The listing builds one solid part. Answer for the finished solid, in the listing's coordinates (mm). Face numbers are marked on the shaded views. A direction names the side the tool comes from. Coordinates: 2 decimals unless noted, no trailing zeros. Loops run counter-clockwise (first coordinate to the right, second up) from the corner with the lowest first, then second, coordinate; pieces in that order, holes last. Notation, with made-up numbers: M 55,-18.5 L 73,-18.5 A16 ccw 73,-0.5 Z; hole C 70,1.5 d4. An arc over 180 degrees is marked long. Answer as a JSON object with one key per item and string values. Group by question number.
1. A cutting plane is placed at C-C on z = 16. State how many separate pieces and enclosed holes the cut face has, and give its area (3 significant figures).
2. Straight lines are drawn through the part: L1, parallel to X at y = -4.5, z = 17; L2, parallel to X at y = -2.3, z = 17; L3, parallel to Z at x = 8, y = -1.95. For each, find the intervals that lie inside material, in ascending order.
3. A cutting plane is placed at A-A on z = 2.25. Give the vertices of the cut face in (x, y).
4. A cutting plane is placed at D-D on y = 7. Give the vertices of the cut face in (x, z).
5. A cutting plane is placed at B-B on x = 31. Give the vertices of the cut face in (y, z), and give its area (3 significant figures).
6. For the marked faces 1 and 2, determine the directions among +Z, -Z, +X, -X, +Y, -Y from which every point of the face is accessible in a straight line to the end or side of a thin tool.
7. Determine the mould class of the marked faces 3, 4, 5 and 6 for opening direction Y: released by +Y, released by -Y, zero draft, split by the parting line, or undercut.
8. Given pin 1 (3.5 mm diameter, centred on x = 46.52, z = 17, fed in from +Y); pin 2 (5 mm diameter, centred on x = 8, z = 17, fed in from +Y); pin 3 (1 mm diameter, centred on y = 9.5, z = 5, fed in from -X); pin 4 (7 mm diameter, centred on x = 46.52, z = 17, fed in from +Y), each flat-ended and moving along its own axis, determine where each tip first touches the part or whether it passes through.
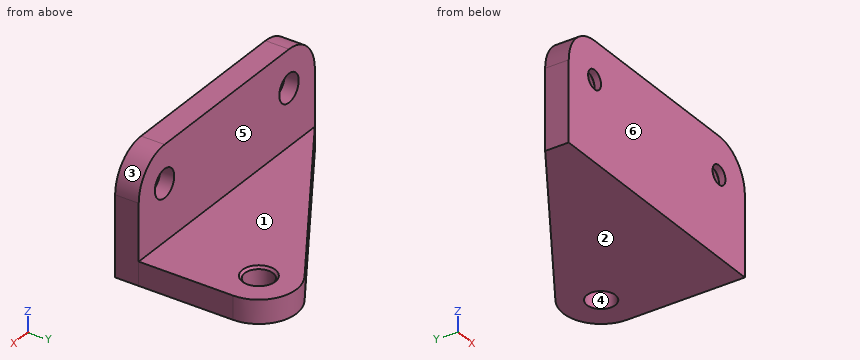
Autodesk Inventor part; units mm, degrees
ref_plane "YZ Plane" through (0, 0, 0) normal (1, 0, 0) x (0, 1, 0)
ref_plane "XZ Plane" through (0, 0, 0) normal (0, 1, 0) x (-1, 0, 0)
ref_plane "XY Plane" through (0, 0, 0) normal (0, 0, 1) x (1, 0, 0)
sketch "Boceto1" plane through (0, 0, 0) normal (0, 0, 1) x (1, 0, 0)
  circle A0 centre (46.519, 19.9996) radius 3
  arc A1 (54.519, 20) -> (42.2378, 26.7576) centre (46.519, 19.9996) ccw
  line L0 (54.52, 0) -> (54.519, 20)
  line L1 (0, 0) -> (42.2378, 26.7576)
  line L2 (0, 0) -> (0, -5)
  line L3 (0, -5) -> (54.52, -5)
  line L4 (54.52, -5) -> (54.52, 0)
  dimension "d5" = 50
  dimension "d6" = 20
  dimension "d8" = 5
  dimension "d9" = 54.52
extrude "Extrusión1" add sketch "Boceto1" along normal blind 5
sketch "Boceto2" plane through (0, 0, 5) normal (0, 0, 1) x (1, 0, 0)
  line L0 (0, 0) -> (0, -5)
  line L1 (0, 0) -> (0, -5)
  line L2 (0, -5) -> (54.52, -5)
  line L3 (0, -5) -> (54.52, -5)
  line L4 (54.52, -5) -> (54.52, 0)
  line L5 (54.52, -5) -> (54.52, 0)
  line L6 (54.52, 0) -> (0, 0)
extrude "Extrusión2" add sketch "Boceto2" along normal blind 20
fillet "Empalme1" radius 8 2 edges at (54.52, -2.5, 25) (0, -2.5, 25)
sketch "Boceto3" plane through (0, 0, 5) normal (0, 1, 0) x (1, 0, 0)
  circle A0 centre (8, -12) radius 3
  circle A1 centre (46.52, -12) radius 3
  point P0 (0, 5)
  dimension "d15" = 6
  dimension "d16" = 6
hole "Agujero1" at (8, 0, 17) at (46.52, 0, 17) direction (0, -1, 0) diameter 6 depth 3 tip angle 118
sketch "Boceto4" plane through (0, 0, 5) normal (0, 1, 0) x (1, 0, 0)
  circle A0 centre (8, -12) radius 3
  circle A1 centre (46.52, -12) radius 3
  point P0 (0, 5)
hole "Agujero2" at (46.52, 0, 17) at (8, 0, 17) direction (0, -1, 0) diameter 4 depth 5 tip angle 118
chamfer "Chaflán1" distance 0.5 angle 45 1 edges at (43.519, 19.9996, 5) measured on face at (33.1116, 5.8435, 5)
properties material "Cobre"
From the geometry:
{
 "1": {"separate pieces": "3", "enclosed holes": "0", "area": "223 mm²"},
 "2": {"L1": "x = 0 to 6, 10 to 44.52, 48.52 to 54.52", "L2": "x = 0 to 5, 11 to 43.52, 49.52 to 54.52", "L3": "z = 0 to 14, 20 to 25"},
 "3": {"outline": "M 0,-5 L 54.52,-5 L 54.52,0 L 54.52,20 A8 ccw 42.24,26.76 L 0,0 Z; hole C 46.52,20 d6"},
 "4": {"outline": "M 11.05,0 L 54.52,0 L 54.52,5 L 11.05,5 Z"},
 "5": {"outline": "M -5,0 L 19.64,0 L 19.64,5 L 0,5 L 0,25 L -5,25 Z", "area": "223 mm²"},
 "6": {"face 1": "+Z, +X, -X, +Y", "face 2": "-Z, +X, -X, +Y, -Y"},
 "7": {"face 3": "zero draft", "face 4": "undercut", "face 5": "released by +Y", "face 6": "released by -Y"},
 "8": {"pin 1": "passes through", "pin 2": "stops at y = -3.3", "pin 3": "stops at x = 14.21", "pin 4": "stops at y = 0"}
}
